Read the model definition and answer for the solid it produces. Units are mm, in the model's axes. Face numbers are marked on the shaded views. Coordinates: 2 decimals unless noted, no trailing zeros. Order: outer loops, then holes, each group sorted by start corner. A loop starts at its lowest first (then second) coordinate and runs counter-clockwise, first axis right, second up.
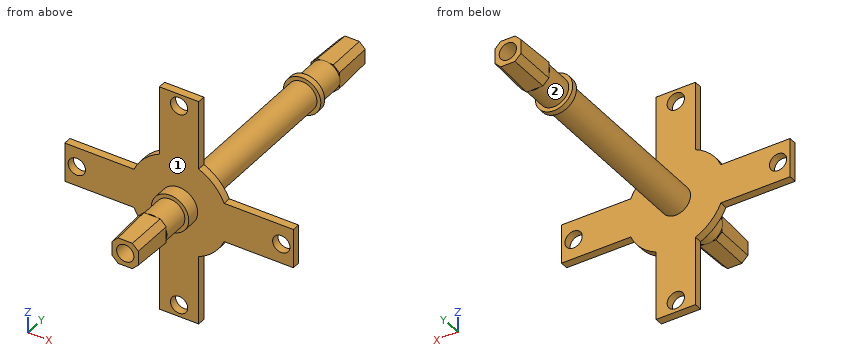
```python
from build123d import *

# Parameters (mm, degrees)
F3_W      = 14.3
F3_H      = 14.3
F4_W      = 13.3
F4_H      = 13.3
F8_SIZE   = 3
F9_R      = 7.5
F10_DEPTH = 135
F11_START = -14
F9_R_2    = 9.5
F11_DEPTH = 11
F12_START = -117
F12_DEPTH = 3
F13_R     = 9.5
F14_DEPTH = 4
F15_D     = 8.8
F16_D     = 8.8


with BuildPart() as f7:
    # F3 (on Front) → F7 section 0
    with BuildSketch(Plane.XZ):
        with Locations((-109.1235904219, 0)):
            Rectangle(F3_W, F3_H)
    # F4 (on offset) → F7 section 1
    with BuildSketch(Plane.XZ.offset(21)):
        with Locations((-109.1235904219, 0)):
            Rectangle(F4_W, F4_H)
    loft()

    # F8
    f8_edges = [f7.edges().sort_by_distance(p)[0] for p in [
        (-116.02359, -10.5, 6.9),
        (-116.02359, -10.5, -6.9),
        (-102.22359, -10.5, 6.9),
        (-102.22359, -10.5, -6.9),
    ]]
    chamfer(f8_edges, length=F8_SIZE)

    # F16 (through all)
    with Locations(Plane.XZ.offset(21)):
        with Locations((-109.1235904219, 0)):
            Hole(F16_D / 2)



with BuildPart() as f10:
    # F9 (on Front) → F10 (new body, through all)
    with BuildSketch(Plane.XZ):
        with Locations((-109.1235904219, 0)):
            Circle(F9_R)
    extrude(amount=-F10_DEPTH)

    # F9 (on Front) → F11 (join)
    with BuildSketch(Plane.XZ.offset(F11_START)):
        with Locations((-109.1235904219, 0)):
            Circle(F9_R_2)
        with Locations((-109.1235904219, 0)):
            Circle(F9_R, mode=Mode.SUBTRACT)
    extrude(amount=-F11_DEPTH)

    # F9 (on Front) → F12 (join)
    with BuildSketch(Plane.XZ.offset(F12_START)):
        with Locations((-109.1235904219, 0)):
            Circle(F9_R_2)
        with Locations((-109.1235904219, 0)):
            Circle(F9_R, mode=Mode.SUBTRACT)
    extrude(amount=-F12_DEPTH)

    # F13 (on face) → F14 (join)
    with BuildSketch(Plane(origin=(0, 25, 0), x_dir=(-1, 0, 0), z_dir=(0, 1, 0))):
        with BuildLine():
            Line((119.1235904219, 22.9128784748), (119.1235904219, 58.1463670404))
            Line((119.1235904219, 58.1463670404), (99.1235904219, 58.1463670404))
            Line((99.1235904219, 58.1463670404), (99.1235904219, 22.9128784748))
            ThreePointArc((99.1235904219, 22.9128784748), (109.1235904219, 25), (119.1235904219, 22.9128784748))
        make_face()
        with BuildLine():
            Line((99.1235904219, -58.1463670404), (119.1235904219, -58.1463670404))
            Line((119.1235904219, -58.1463670404), (119.1235904219, -22.9128784748))
            ThreePointArc((119.1235904219, -22.9128784748), (109.1235904219, -25), (99.1235904219, -22.9128784748))
            Line((99.1235904219, -22.9128784748), (99.1235904219, -58.1463670404))
        make_face()
        with BuildLine():
            Line((167.2699574623, -10), (167.2699574623, 10))
            Line((167.2699574623, 10), (132.0364688967, 10))
            ThreePointArc((132.0364688967, 10), (133.5962482452, 5.1077410922), (134.1235904219, 0))
            ThreePointArc((134.1235904219, 0), (133.5962482452, -5.1077410922), (132.0364688967, -10))
            Line((132.0364688967, -10), (167.2699574623, -10))
        make_face()
        with BuildLine():
            ThreePointArc((134.1235904219, 0), (133.5962482452, 5.1077410922), (132.0364688967, 10))
            ThreePointArc((132.0364688967, 10), (126.8012599516, 17.6776695297), (119.1235904219, 22.9128784748))
            Line((119.1235904219, 22.9128784748), (99.1235904219, 22.9128784748))
            ThreePointArc((99.1235904219, 22.9128784748), (91.4459208923, 17.6776695297), (86.2107119471, 10))
            ThreePointArc((86.2107119471, 10), (84.1235904219, 0), (86.2107119471, -10))
            ThreePointArc((86.2107119471, -10), (91.4459208923, -17.6776695297), (99.1235904219, -22.9128784748))
            ThreePointArc((99.1235904219, -22.9128784748), (109.1235904219, -25), (119.1235904219, -22.9128784748))
            ThreePointArc((119.1235904219, -22.9128784748), (126.8012599516, -17.6776695297), (132.0364688967, -10))
            ThreePointArc((132.0364688967, -10), (133.5962482452, -5.1077410922), (134.1235904219, 0))
        make_face()
        with Locations((109.1235904219, 0)):
            Circle(F13_R, mode=Mode.SUBTRACT)
        with BuildLine():
            Line((86.2107119471, 10), (50.9772233815, 10))
            Line((50.9772233815, 10), (50.9772233815, -10))
            Line((50.9772233815, -10), (86.2107119471, -10))
            ThreePointArc((86.2107119471, -10), (84.1235904219, 0), (86.2107119471, 10))
        make_face()
        with BuildLine():
            Line((99.1235904219, 22.9128784748), (119.1235904219, 22.9128784748))
            ThreePointArc((119.1235904219, 22.9128784748), (109.1235904219, 25), (99.1235904219, 22.9128784748))
        make_face()
    extrude(amount=-F14_DEPTH)

    # F15 (through all)
    with Locations(Plane(origin=(0, 25, 0), x_dir=(-1, 0, 0), z_dir=(0, 1, 0))):
        with Locations((109.1235904219, 52), (57.1235904219, 0), (161.1235904219, 0), (109.1235904219, -52)):
            Hole(F15_D / 2)


with BuildPart() as f7_1:
    add(f7.part)

    add(f10.part)  # F17 merges F10
    # F17: F7 across plane
    add(f7.part.mirror(Plane.XZ.offset(-67.5)))


solid = f7_1.part
```
1) A cutting plane is placed at C-C, the plane x = -145.5. Determine the outline of the cut face in (y, z), and give its area (3 significant figures).
A:
outline: (21, -10) - (25, -10) - (25, 10) - (21, 10) - close
area: 80.0 mm2
2) A cutting plane is placed at D-D, the plane y = 76.5. Determine the outline of the cut face in (x, z).
A:
outline: circle Ø15 at (-109.12, 0)
3) A cutting plane is placed at A-A, the plane z = 52. Determine the outline of the cut face in (x, y), and give its area (3 significant figures).
A:
outline: (-119.12, 21) - (-113.52, 21) - (-113.52, 25) - (-119.12, 25) - close; (-104.72, 21) - (-99.12, 21) - (-99.12, 25) - (-104.72, 25) - close
area: 44.8 mm2
4) A cutting plane is placed at B-B, the plane z = 0. State how many separate pieces and enclosed holes the cut face has, and give its area (3 significant figures).
A:
separate pieces: 3
enclosed holes: 0
area: 2,610 mm2
5) Flat-ended cylindrical pins translate along their axes: pin 1 Ø3 at (y, z) = (22.5, -49) entering from -X; pin 2 Ø1.5 at (x, y) = (-111.5, 32) entering from +Z; pin 3 Ø2 at (x, y) = (-147.5, 22.5) entering from -Z. Find the tip coordinate at first contact, or state that the pin passes through.
A:
pin 1: stops at x = -119.12
pin 2: stops at z = 7.32
pin 3: stops at z = -10
6) Straight lines are drawn through the part: line 1 (Y direction, x = -75.5, z = 8.5); line 2 (Z direction, x = -102.5, y = -10); line 3 (Z direction, x = -117.5, y = 20.5). For each, find the intervals that lie inside material, in ascending order.
A:
line 1: y = 21 to 25
line 2: z = -4.2 to 4.2
line 3: z = -4.48 to 4.48
7) Determine the mould class of the marked faces 1 and 2 for opening direction Y: pulls with the +Y half, pulls with the -Y half, needs draft (parallel to the pull), parting line crosses it, or undercut.
A:
face 1: pulls with the -Y half
face 2: undercut
